```python
from build123d import *

# Parameters (mm, degrees)
F1_DEPTH = 25
F2_R     = 16.943766
F3_DEPTH = 20


with BuildPart() as f1:
    # F0 (on Front) → F1 (new body)
    with BuildSketch(Plane.XZ):
        with BuildLine():
            Line((25.009147, 19.70269), (-16.551667, 29.257499))
            ThreePointArc((-16.551667, 29.257499), (-53.298677, 0), (-16.551667, -29.257499))
            Line((-16.551667, -29.257499), (25.009147, -19.70269))
            ThreePointArc((25.009147, -19.70269), (40.696177, 0), (25.009147, 19.70269))
        make_face()
    extrude(amount=-F1_DEPTH)

    # F2 (on face) → F3 (cut)
    with BuildSketch(Plane.XZ):
        with Locations((-23.27795, 0)):
            Circle(F2_R)
    extrude(amount=-F3_DEPTH, mode=Mode.SUBTRACT)


solid = f1.part
```
The model under review builds one solid part; all positions refer to its coordinate system, in mm. A direction names the side the tool comes from. Round coordinates to 2 decimals unless told otherwise and drop trailing zeros. Order: outer loops, then holes, each group sorted by start corner. A loop starts at its lowest first (then second) coordinate and runs counter-clockwise, first axis right, second up. Notation, with made-up numbers: M -18.75,-1 L 29.25,-1 A25 cw 29.25,11 Z; hole C 89.25,25.25 d6. An arc over 180 degrees is marked long. Use a Markdown table: item, result.
1) Consider section D-D (x = 5). Write out the cut boundary in (y, z), then the cut area to 3 significant figures.
Report:
| item | result |
|---|---|
| outline | M 0,-24.3 L 25,-24.3 L 25,24.3 L 0,24.3 Z |
| area | 1,220 mm^2 |
2) Draft analysis for pull direction Z (two halves, no side actions). For faces 3 (the face through (40.693, 12.325, -0.381)), 4 (the face through (-26.95, 9.86, -16.54)), 5 (the face through (3.938, 12.325, -24.547)), state which applies: released by +Z, released by -Z, zero draft, split by the parting line, or undercut.
Report:
| item | result |
|---|---|
| face 3 | split by the parting line |
| face 4 | undercut |
| face 5 | released by -Z |
3) Consider section A-A (y = 13.75). Write out the cut boundary in (x, z), then the cut area to 3 significant figures.
Report:
| item | result |
|---|---|
| outline | M -16.55,-29.26 L 25.01,-19.7 A20.22 ccw 25.01,19.7 L -16.55,29.26 A30.02 ccw long Z; hole C -23.28,0 d33.89 |
| area | 3,410 mm^2 |
4) Consider section C-C (y = 22.25). Write out the cut boundary in (x, z), then the cut area to 3 significant figures.
Report:
| item | result |
|---|---|
| outline | M -16.55,-29.26 L 25.01,-19.7 A20.22 ccw 25.01,19.7 L -16.55,29.26 A30.02 ccw long Z |
| area | 4,310 mm^2 |
5) Insertion check: pin 1 (8 mm diameter, centred on y = 3.5, z = 19.5, fed in from +X); pin 2 (1.5 mm diameter, centred on x = 25, y = 12.5, fed in from +Z); pin 3 (3 mm diameter, centred on y = 10.5, z = -9, fed in from -X). Each pin has a flat end and moves straight along its axis. Give the tip position at first contact, or say it passes through.
Report:
| item | result |
|---|---|
| pin 1 | x = 33.46 |
| pin 2 | z = 19.88 |
| pin 3 | x = -52.35 |
6) Wall thickness on line 1 along Z through (x, y) = (-14.5, 19); line 2 along Z through (x, y) = (-35.5, 18.25); line 3 along X through (y, z) = (2, 1): over which ranges is each line inside the solid? List them lowest first. Write a range as [from, to].
Report:
| item | result |
|---|---|
| line 1 | [-28.79, -14.49], [14.49, 28.79] |
| line 2 | [-27.42, -11.74], [11.74, 27.42] |
| line 3 | [-53.28, -40.19], [-6.36, 40.67] |
7) Tool access review of faces 1 (the face through (-24, 20, 0)), 2 (the face through (-7, 25, 0)): name each direction out of +Z, -Z, +X, -X, +Y, -Y from which nothing blocks a thin tool from reaching the whole face with its end or side.
Report:
| item | result |
|---|---|
| face 1 | -Y |
| face 2 | +Z, -Z, +X, -X, +Y |
8) Consider section B-B (z = 0). Write out the cut boundary in (x, y), then the cut area to 3 significant figures.
Report:
| item | result |
|---|---|
| outline | M -53.3,0 L -40.22,0 L -40.22,20 L -6.33,20 L -6.33,0 L 40.7,0 L 40.7,25 L -53.3,25 Z |
| area | 1,670 mm^2 |
